Input: part model. Units: mm. Frame: model coordinates. A direction names the side the tool comes from. Coordinates: 2 decimals unless noted, no trailing zeros. Write each loop counter-clockwise with the first axis right and the second up, starting at its lowest first coordinate (ties: lowest second). Pieces come first, ordered by that corner, then holes. Notation, with made-up numbers: (1.25, -39.75) - (16.25, -39.75) arc R35 cw to (16.25, -4.75) - close; hole circle Ø1 at (13, 18). An arc over 180 degrees is marked (long way). One line per question, with ' | ' between items. Start each with the question number.
1) Section query B-B on y = 58.5. Return loops of the section in (x, z).
2) First-contact query: P1, Ø5, axis at y = -57, z = 6.5, coming from the -X side; P2, Ø1.5, axis at y = 53, z = 7, coming from the +X side; P3, Ø6, axis at y = 19.5, z = 5.5, coming from the +X side; P4, Ø4.5, axis at x = 56.47, y = -50.02, coming from the -Z side. Flat tips, straight axial feed; report the tip coordinate or a pass-through.
3) Reachability of faces 4 (the flat face through (-54.286, 55, 6)), 5 (the cylindrical face through (158.517, -40.592, 6.439)) from +Z, -Z, +X, -X, +Y, -Y: full face, straight path, thin tool, end or side. Return the list, or none.
4) Line query: line 1 (X direction, y = -51.5, z = 5.5); line 2 (Y direction, x = 112.5, z = 9.5); line 3 (X direction, y = 55, z = 8.25). Output: solid intervals per line, ascending.
5) Section query A-A on x = 39.5. Return loops of the section in (y, z), and give its area (3 significant figures).
6) Draft query along Y for faces 1 (the cylindrical face through (-57.29, 90.12, 6.44)), 2 (the cylindrical face through (117.776, -39.823, 6.439)), 3 (the flat face through (15, -39, 12.7)). Return one class per face: released by +Y, released by -Y, zero draft, split by the parting line, or undercut.
```python
from build123d import *

# Parameters (mm, degrees)
RESSALTO_EXTRUS_O1_DEPTH   = 12.7
CIRCULO_DE_ROLAMENTO_REACH = 245.52
ESBO_O3_R                  = 16
CORTE_EXTRUS_O3_REACH      = 245.52
ESBO_O5_R                  = 3
ESBO_O6_R                  = 2.5
CORTE_EXTRUS_O4_DEPTH      = 30
CORTE_EXTRUS_O6_REACH      = 245.52
CORTE_EXTRUS_O7_REACH      = 245.52
ESBO_O10_R                 = 2.78
CORTE_EXTRUS_O8_REACH      = 245.52
ESBO_O12_R                 = 2.6
FILETE1_R                  = 10


with BuildPart() as part:
    # Esboço1 → Ressalto-extrusão1 (new body)
    with BuildSketch(Plane.XY):
        Polygon((-114.28595772, -92.023971813), (224.71404228, -92.023971813), (224.71404228, -36.023971813), (5.71404228, -36.023971813), (-54.28595772, 23.976028187), (-54.28595772, 92.976028187), (-114.28595772, 92.976028187), align=None)
    extrude(amount=RESSALTO_EXTRUS_O1_DEPTH)

    # Esboço3 → circulo de rolamento (cut, up to next)
    with BuildSketch(Plane.XY.offset(12.7), mode=Mode.PRIVATE) as circulo_de_rolamento_sk1:
        with Locations((138.21404228, -64.023971813)):
            Circle(ESBO_O3_R)
    circulo_de_rolamento_tool1 = extrude(circulo_de_rolamento_sk1.sketch, amount=-CIRCULO_DE_ROLAMENTO_REACH, mode=Mode.PRIVATE) & part.part
    add(circulo_de_rolamento_tool1.solids().sort_by_distance((138.214042, -64.023972, 12.7))[0], mode=Mode.SUBTRACT)

    # Esboço5 → Corte-extrusão3 (cut, up to next)
    with BuildSketch(Plane.XY.offset(12.7), mode=Mode.PRIVATE) as corte_extrus_o3_sk1:
        with Locations((114.91404228, -40.723971813)):
            Circle(ESBO_O5_R)
    corte_extrus_o3_tool1 = extrude(corte_extrus_o3_sk1.sketch, amount=-CORTE_EXTRUS_O3_REACH, mode=Mode.PRIVATE) & part.part
    # Esboço5 → Corte-extrusão3 (cut, up to next)
    with BuildSketch(Plane.XY.offset(12.7), mode=Mode.PRIVATE) as corte_extrus_o3_sk2:
        with Locations((161.51404228, -40.723971813)):
            Circle(ESBO_O5_R)
    corte_extrus_o3_tool2 = extrude(corte_extrus_o3_sk2.sketch, amount=-CORTE_EXTRUS_O3_REACH, mode=Mode.PRIVATE) & part.part
    # Esboço5 → Corte-extrusão3 (cut, up to next)
    with BuildSketch(Plane.XY.offset(12.7), mode=Mode.PRIVATE) as corte_extrus_o3_sk3:
        with Locations((161.51404228, -87.323971813)):
            Circle(ESBO_O5_R)
    corte_extrus_o3_tool3 = extrude(corte_extrus_o3_sk3.sketch, amount=-CORTE_EXTRUS_O3_REACH, mode=Mode.PRIVATE) & part.part
    # Esboço5 → Corte-extrusão3 (cut, up to next)
    with BuildSketch(Plane.XY.offset(12.7), mode=Mode.PRIVATE) as corte_extrus_o3_sk4:
        with Locations((114.91404228, -87.323971813)):
            Circle(ESBO_O5_R)
    corte_extrus_o3_tool4 = extrude(corte_extrus_o3_sk4.sketch, amount=-CORTE_EXTRUS_O3_REACH, mode=Mode.PRIVATE) & part.part
    add(corte_extrus_o3_tool1.solids().sort_by_distance((114.914042, -40.723972, 12.7))[0], mode=Mode.SUBTRACT)
    add(corte_extrus_o3_tool2.solids().sort_by_distance((161.514042, -40.723972, 12.7))[0], mode=Mode.SUBTRACT)
    add(corte_extrus_o3_tool3.solids().sort_by_distance((161.514042, -87.323972, 12.7))[0], mode=Mode.SUBTRACT)
    add(corte_extrus_o3_tool4.solids().sort_by_distance((114.914042, -87.323972, 12.7))[0], mode=Mode.SUBTRACT)

    # Esboço6 → Corte-extrusão4 (cut)
    with BuildSketch(Plane.ZY.offset(114.28595772)):
        with Locations(Location((4.765, 67.976028187, 0), (0, 0, 270))):
            Circle(ESBO_O6_R)
        with Locations(Location((4.765, 42.976028187, 0), (0, 0, 270))):
            Circle(ESBO_O6_R)
        with Locations(Location((4.765, 17.976028187, 0), (0, 0, 270))):
            Circle(ESBO_O6_R)
    extrude(amount=-CORTE_EXTRUS_O4_DEPTH, mode=Mode.SUBTRACT)

    # Esboço9 → Corte-extrusão6 (cut, up to next)
    with BuildSketch(Plane.XY.offset(12.7), mode=Mode.PRIVATE) as corte_extrus_o6_sk1:
        Polygon((-29.28595772, -92.023971813), (-114.28595772, -7.023971813), (-114.28595772, -92.023971813), align=None)
    corte_extrus_o6_tool1 = extrude(corte_extrus_o6_sk1.sketch, amount=-CORTE_EXTRUS_O6_REACH, mode=Mode.PRIVATE) & part.part
    add(corte_extrus_o6_tool1.solids().sort_by_distance((-85.952624, -63.690638, 12.7))[0], mode=Mode.SUBTRACT)

    # Esboço10 → Corte-extrusão7 (cut, up to next)
    with BuildSketch(Plane.XY.offset(12.7), mode=Mode.PRIVATE) as corte_extrus_o7_sk1:
        with Locations((56.47404228, -50.023971813)):
            Circle(ESBO_O10_R)
    corte_extrus_o7_tool1 = extrude(corte_extrus_o7_sk1.sketch, amount=-CORTE_EXTRUS_O7_REACH, mode=Mode.PRIVATE) & part.part
    # Esboço10 → Corte-extrusão7 (cut, up to next)
    with BuildSketch(Plane.XY.offset(12.7), mode=Mode.PRIVATE) as corte_extrus_o7_sk2:
        with Locations((56.47404228, -64.023971813)):
            Circle(ESBO_O10_R)
    corte_extrus_o7_tool2 = extrude(corte_extrus_o7_sk2.sketch, amount=-CORTE_EXTRUS_O7_REACH, mode=Mode.PRIVATE) & part.part
    # Esboço10 → Corte-extrusão7 (cut, up to next)
    with BuildSketch(Plane.XY.offset(12.7), mode=Mode.PRIVATE) as corte_extrus_o7_sk3:
        with Locations((56.47404228, -78.023971813)):
            Circle(ESBO_O10_R)
    corte_extrus_o7_tool3 = extrude(corte_extrus_o7_sk3.sketch, amount=-CORTE_EXTRUS_O7_REACH, mode=Mode.PRIVATE) & part.part
    add(corte_extrus_o7_tool1.solids().sort_by_distance((56.474042, -50.023972, 12.7))[0], mode=Mode.SUBTRACT)
    add(corte_extrus_o7_tool2.solids().sort_by_distance((56.474042, -64.023972, 12.7))[0], mode=Mode.SUBTRACT)
    add(corte_extrus_o7_tool3.solids().sort_by_distance((56.474042, -78.023972, 12.7))[0], mode=Mode.SUBTRACT)

    # Esboço12 → Corte-extrusão8 (cut, up to next)
    with BuildSketch(Plane.XY.offset(12.7), mode=Mode.PRIVATE) as corte_extrus_o8_sk1:
        with Locations((219.95404228, -50.023971813)):
            Circle(ESBO_O12_R)
    corte_extrus_o8_tool1 = extrude(corte_extrus_o8_sk1.sketch, amount=-CORTE_EXTRUS_O8_REACH, mode=Mode.PRIVATE) & part.part
    # Esboço12 → Corte-extrusão8 (cut, up to next)
    with BuildSketch(Plane.XY.offset(12.7), mode=Mode.PRIVATE) as corte_extrus_o8_sk2:
        with Locations((219.95404228, -64.023971813)):
            Circle(ESBO_O12_R)
    corte_extrus_o8_tool2 = extrude(corte_extrus_o8_sk2.sketch, amount=-CORTE_EXTRUS_O8_REACH, mode=Mode.PRIVATE) & part.part
    # Esboço12 → Corte-extrusão8 (cut, up to next)
    with BuildSketch(Plane.XY.offset(12.7), mode=Mode.PRIVATE) as corte_extrus_o8_sk3:
        with Locations((219.95404228, -78.023971813)):
            Circle(ESBO_O12_R)
    corte_extrus_o8_tool3 = extrude(corte_extrus_o8_sk3.sketch, amount=-CORTE_EXTRUS_O8_REACH, mode=Mode.PRIVATE) & part.part
    add(corte_extrus_o8_tool1.solids().sort_by_distance((219.954042, -50.023972, 12.7))[0], mode=Mode.SUBTRACT)
    add(corte_extrus_o8_tool2.solids().sort_by_distance((219.954042, -64.023972, 12.7))[0], mode=Mode.SUBTRACT)
    add(corte_extrus_o8_tool3.solids().sort_by_distance((219.954042, -78.023972, 12.7))[0], mode=Mode.SUBTRACT)

    # Filete1
    filete1_edges = [part.edges().sort_by_distance(p)[0] for p in [
        (-54.28595772, 92.976028187, 6.35),
        (-54.28595772, 23.976028187, 6.35),
        (5.71404228, -36.023971813, 6.35),
        (-29.28595772, -92.023971813, 6.35),
    ]]
    fillet(filete1_edges, radius=FILETE1_R)


solid = part.part
```
Answer key:
1) outline: (-114.29, 0) - (-54.29, 0) - (-54.29, 12.7) - (-114.29, 12.7) - close
2) P1: x = -66.81 | P2: x = -54.29 | P3: x = -46.81 | P4: through
3) face 4: +Z, -Z, +X, +Y | face 5: +Z, -Z
4) line 1: -69.81 to 54.12, 58.83 to 128.26, 148.17 to 217.81, 222.09 to 224.71 | line 2: -92.02 to -89.11, -85.54 to -42.51, -38.94 to -36.02 | line 3: -114.29 to -54.29
5) outline: (-92.02, 0) - (-36.02, 0) - (-36.02, 12.7) - (-92.02, 12.7) - close | area: 711 mm²
6) face 1: released by +Y | face 2: undercut | face 3: zero draft
